Verification items for this drawing (mm, ordinates from the low corner). A direction names the side the tool comes from. Coordinates: 2 decimals unless noted, no trailing zeros. Loops run counter-clockwise (first coordinate to the right, second up) from the corner with the lowest first, then second, coordinate; pieces in that order, holes last. Notation, with made-up numbers: M 34.5,29 L 58.5,29 A22 ccw 58.5,60 Z; hole C 72.25,67.5 d4. An arc over 180 degrees is marked long. One line per question, with ' | ' between items. Start each with the question number.
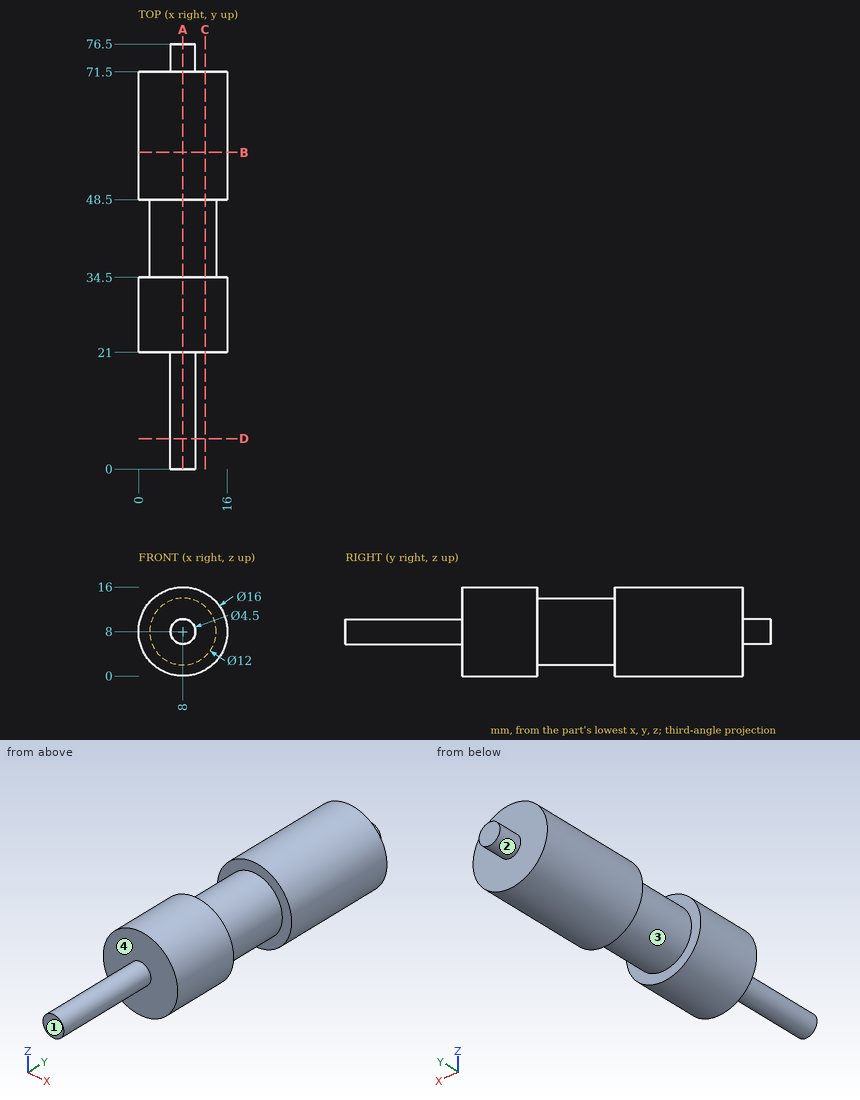
1. Sectioned sample at D-D (y = 5.5). Record the cut outline in (x, z), and give its area (3 significant figures).
2. Tool access check on the marked faces 1, 2, 3 and 4. Record the directions out of +Z, -Z, +X, -X, +Y, -Y that give a thin tool (end or side, any length) a straight path to the whole face; none if there is none.
3. Depth check by flat-ended pin: pin 1 Ø1 at (x, z) = (4, 11.5) entering from -Y; pin 2 Ø8 at (y, z) = (41.5, 6) entering from +X; pin 3 Ø2 at (y, z) = (63, 9.5) entering from +X. Enter the tip coordinate at first touch or a pass-through.
4. Thickness scan on line 1 (Y direction, x = 15.25, z = 9); line 2 (X direction, y = 61, z = 7.5); line 3 (Y direction, x = 12.5, z = 4.75). Record the ranges inside material, lowest first.
5. Sectioned sample at C-C (x = 12). Record the cut outline in (y, z), and give its area (3 significant figures).
6. Sectioned sample at A-A (x = 8). Record the cut outline in (y, z).
7. Sectioned sample at B-B (y = 57). Record the cut outline in (x, z).
Result:
1) outline: C 8,8 d4.5 | area: 15.9 mm2
2) face 1: +Z, -Z, +X, -X, -Y | face 2: +Y | face 3: none | face 4: -Y
3) pin 1: stops at y = 21 | pin 2: stops at x = 14 | pin 3: stops at x = 15.98
4) line 1: y = 21 to 34.5, 48.5 to 71.5 | line 2: x = 0.02 to 15.98 | line 3: y = 21 to 71.5
5) outline: M 21,1.07 L 34.5,1.07 L 34.5,3.53 L 48.5,3.53 L 48.5,1.07 L 71.5,1.07 L 71.5,14.93 L 48.5,14.93 L 48.5,12.47 L 34.5,12.47 L 34.5,14.93 L 21,14.93 Z | area: 631 mm2
6) outline: M 0,5.75 L 21,5.75 L 21,0 L 34.5,0 L 34.5,2 L 48.5,2 L 48.5,0 L 71.5,0 L 71.5,5.75 L 76.5,5.75 L 76.5,10.25 L 71.5,10.25 L 71.5,16 L 48.5,16 L 48.5,14 L 34.5,14 L 34.5,16 L 21,16 L 21,10.25 L 0,10.25 Z
7) outline: C 8,8 d16
